Part model, mm, in its own coordinate system. Round coordinates to 2 decimals unless told otherwise and drop trailing zeros. Write each loop counter-clockwise with the first axis right and the second up, starting at its lowest first coordinate (ties: lowest second). Pieces come first, ordered by that corner, then holes.
```python
from build123d import *

# Parameters (mm, degrees)
BOSS_EXTRUDE1_DEPTH = 3.175
SKETCH2_R           = 1.4732
CUT_EXTRUDE1_DEPTH  = 4.175
CUT_EXTRUDE2_DEPTH  = 4.175
FILLET1_R           = 3
CUT_EXTRUDE5_DEPTH  = 4.175


with BuildPart() as part:
    # Sketch1 → Boss-Extrude1 (new body)
    with BuildSketch(Plane.XY):
        with BuildLine():
            Line((12.587486719, 44.5), (42.587486719, 44.5))
            ThreePointArc((42.587486719, 44.5), (61.594999998, 0), (42.587486719, -44.5))
            Line((42.587486719, -44.5), (12.587486719, -44.5))
            Line((12.587486719, -44.5), (12.587486719, 44.5))
        make_face()
    extrude(amount=BOSS_EXTRUDE1_DEPTH)

    # Sketch2 → Cut-Extrude1 (cut, through all)
    with BuildSketch(Plane.XY.offset(3.175)):
        with Locations((16.354311186, -40.81189221)):
            Circle(SKETCH2_R)
        with Locations((35.404311186, -40.81189221)):
            Circle(SKETCH2_R)
        with Locations((16.354311186, 40.81189221)):
            Circle(SKETCH2_R)
        with Locations((35.404311186, 40.81189221)):
            Circle(SKETCH2_R)
    extrude(amount=-CUT_EXTRUDE1_DEPTH, mode=Mode.SUBTRACT)

    # Sketch3 → Cut-Extrude2 (cut, through all)
    with BuildSketch(Plane.XY.offset(3.175)):
        with BuildLine():
            Line((58.42, 7.62), (61.121842452, 7.62))
            ThreePointArc((61.121842452, 7.62), (61.594999998, 0), (61.121842452, -7.62))
            Line((61.121842452, -7.62), (58.42, -7.62))
            Line((58.42, -7.62), (58.42, 7.62))
        make_face()
    extrude(amount=-CUT_EXTRUDE2_DEPTH, mode=Mode.SUBTRACT)

    # Fillet1
    fillet1_edges = [part.edges().sort_by_distance(p)[0] for p in [
        (12.587486719, 44.5, 1.5875),
        (42.587486719, 44.5, 1.5875),
        (42.587486719, -44.5, 1.5875),
        (12.587486719, -44.5, 1.5875),
    ]]
    fillet(fillet1_edges, radius=FILLET1_R)

    # Sketch5 → Cut-Extrude5 (cut, through all)
    with BuildSketch(Plane.XY.offset(3.175)):
        with BuildLine():
            Line((16.612162061, -17.554236987), (48.444763602, -17.554236987))
            ThreePointArc((48.444763602, -17.554236987), (50.390526615, -19.5), (48.444763602, -21.445763013))
            Line((48.444763602, -21.445763013), (16.612162061, -21.445763013))
            ThreePointArc((16.612162061, -21.445763013), (14.666399048, -19.5), (16.612162061, -17.554236987))
        make_face()
    extrude(amount=-CUT_EXTRUDE5_DEPTH, mode=Mode.SUBTRACT)


solid = part.part
```
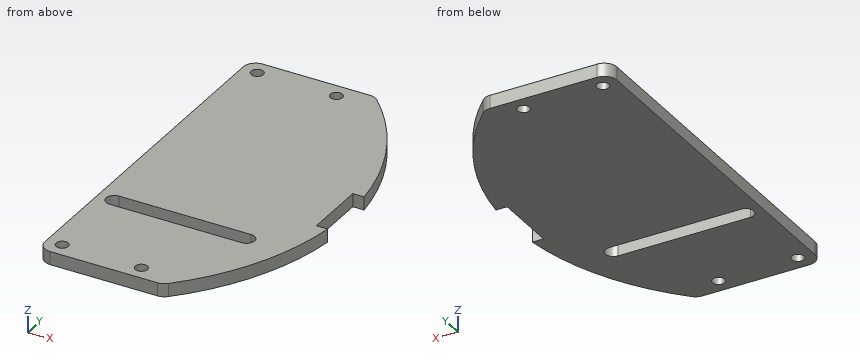
Q1. Cut at B-B on y = -19.5. Write the cut outline in (x, z) (3 decimals), plus the area to 3 significant figures.
Values follow:
outline: (12.587, 0) - (14.666, 0) - (14.666, 3.175) - (12.587, 3.175) - close; (50.391, 0) - (58.427, 0) - (58.427, 3.175) - (50.391, 3.175) - close
area: 32.1 mm2
Q2. Cut at C-C on z = 0.6. Write the cut outline in (x, y) (3 decimals).
Values follow:
outline: (12.587, -41.5) arc R3 ccw to (15.587, -44.5) - (41.366, -44.5) arc R3 ccw to (43.484, -43.625) arc R61.595 ccw to (61.122, -7.62) - (58.42, -7.62) - (58.42, 7.62) - (61.122, 7.62) arc R61.595 ccw to (43.484, 43.625) arc R3 ccw to (41.366, 44.5) - (15.587, 44.5) arc R3 ccw to (12.587, 41.5) - close; hole circle Ø2.946 at (16.354, -40.812); hole circle Ø2.946 at (16.354, 40.812); hole (16.612, -21.446) - (48.445, -21.446) arc R1.946 ccw to (48.445, -17.554) - (16.612, -17.554) arc R1.946 ccw to start; hole circle Ø2.946 at (35.404, -40.812); hole circle Ø2.946 at (35.404, 40.812)
Q3. Cut at A-A on x = 32.5. Write the cut outline in (y, z) (3 decimals).
Values follow:
outline: (-44.5, 0) - (-21.446, 0) - (-21.446, 3.175) - (-44.5, 3.175) - close; (-17.554, 0) - (44.5, 0) - (44.5, 3.175) - (-17.554, 3.175) - close
Q4. Drop a flat-ended pin along its axis: pin 1 (10 mm diameter, centred on x = 51, y = 7.5, fed in from -Z). Give the stop position or say it passes through.
Values follow:
pin 1: stops at z = 0
Q5. Wall check: L1, parallel to Y at x = 37, z = 2.2; L2, parallel to X at y = -41, z = 0.95; L3, parallel to Y at x = 34.5, z = 2.1. Give the ranges that are in metal, low to high.
Values follow:
L1: y = -44.5 to -21.45, -17.55 to 44.5
L2: x = 12.59 to 14.89, 17.82 to 33.94, 36.87 to 45.97
L3: y = -44.5 to -41.97, -39.65 to -21.45, -17.55 to 39.65, 41.97 to 44.5
Q6. Cut at D-D on y = -5. Write the cut outline in (x, z) (3 decimals).
Values follow:
outline: (12.587, 0) - (58.42, 0) - (58.42, 3.175) - (12.587, 3.175) - close
